Autodesk Inventor part; units mm, degrees
ref_plane "YZ Plane" through (0, 0, 0) normal (1, 0, 0) x (0, 1, 0)
ref_plane "XZ Plane" through (0, 0, 0) normal (0, 1, 0) x (-1, 0, 0)
ref_plane "XY Plane" through (0, 0, 0) normal (0, 0, 1) x (1, 0, 0)
sketch "スケッチ1" plane through (0, 0, 0) normal (0, 1, 0) x (-1, 0, 0)
  line L0 (9.5, -10) -> (-9.5, -10)
  line L1 (-9.5, -10) -> (-9.5, 10)
  line L2 (-9.5, 10) -> (9.5, 10)
  line L3 (9.5, 10) -> (9.5, -10)
  line L4 (9.5, -10) -> (-9.5, 10) construction
  point P0 (0, 0)
  point P1 (0, 0)
  dimension "d0" = 19
  dimension "d1" = 20
extrude "押し出し1" add sketch "スケッチ1" along normal blind 1.5
sketch "スケッチ3" plane through (0, 0, 0) normal (0, -1, 0) x (1, 0, 0)
  line L0 (-9.5, 10) -> (9.5, 10)
  line L1 (-9.5, -10) -> (-9.5, 10)
  line L2 (9.5, -10) -> (-9.5, -10)
  line L3 (9.5, 10) -> (9.5, -10)
  line L4 (-9.5, 0) -> (9.5, 0)
  line L5 (-9.5, 10) -> (9.5, 10)
  line L6 (0, 10) -> (0, -10)
  line L7 (0, 2.5) -> (-3.1667, 2.5)
  line L8 (-3.1667, 2.5) -> (-3.1667, 7.5)
  line L9 (-3.1667, 7.5) -> (0, 7.5)
  line L10 (0, 2.5) -> (3.1667, 2.5)
  line L11 (3.1667, 2.5) -> (3.1667, 7.5)
  line L12 (3.1667, 7.5) -> (0, 7.5)
  line L13 (0, -2.5) -> (-3.1667, -2.5)
  line L14 (-3.1667, -2.5) -> (-3.1667, -7.5)
  line L15 (-3.1667, -7.5) -> (0, -7.5)
  line L16 (3.1667, -2.5) -> (3.1667, -7.5)
  line L17 (0, -2.5) -> (3.1667, -2.5)
  line L18 (3.1667, -7.5) -> (0, -7.5)
  point P0 (0, 0)
  point P1 (0, 0)
  dimension "d8" = 3.1667
  dimension "d9" = 2.5
  dimension "d10" = 5
extrude "押し出し2" add sketch "スケッチ3" along normal blind 1.6 contours L12 L11 L10 L6 | L6 L7 L8 L9 | L17 L16 L18 L6 | L6 L15 L14 L13
sketch "スケッチ4" plane through (0, -1.6, 0) normal (0, -1, 0) x (1, 0, 0)
  line L0 (3.1667, 2.5) -> (3.1667, 7.5)
  line L1 (-3.1667, 7.5) -> (-3.1667, 2.5)
  line L2 (-3.1667, -2.5) -> (-3.1667, -7.5)
  line L3 (3.1667, -7.5) -> (3.1667, -2.5)
  line L4 (3.1667, 7.5) -> (3.1667, 2.5) construction
  line L5 (3.1667, 5) -> (6.3333, 5) construction
  line L6 (6.3333, 5) -> (9.5, 5) construction
  line L7 (9.5, 10) -> (9.5, -10) construction
  line L8 (9.5, 0) -> (-9.5, 0)
  line L9 (-9.5, -10) -> (-9.5, 10)
  line L10 (3.1667, 2.5) -> (-3.1667, 2.5)
  line L11 (0, 2.5) -> (0, -2.5)
  point P0 (0, 0)
  point P1 (6.3333, -5)
  point P2 (-6.3333, 5)
  point P3 (-6.3333, -5)
hole "穴1" at (6.3333, -1.6, 5) at (6.3333, -1.6, -5) at (-6.3333, -1.6, 5) at (-6.3333, -1.6, -5) direction (0, 1, 0) diameter 1.567 end through all
fillet "フィレット1" radius 1.5 8 edges at (3.1667, -0.8, 2.5) (3.1667, -0.8, 7.5) (-3.1667, -0.8, 7.5) (-3.1667, -0.8, 2.5) (3.1667, -0.8, -2.5) (3.1667, -0.8, -7.5) (-3.1667, -0.8, -7.5) (-3.1667, -0.8, -2.5)
properties part number "jump" material "ABS プラスチック"
The listing builds one solid part. Answer for the finished solid, in the listing's coordinates (mm). A direction names the side the tool comes from. Give positions to 0.01 mm unless a question says otherwise; leave off trailing zeros. Write each loop counter-clockwise with the first axis right and the second up, starting at its lowest first coordinate (ties: lowest second). Pieces come first, ordered by that corner, then holes. Notation, with made-up numbers: (-35.75, -4.5) - (21.25, -4.5) arc R23 cw to (21.25, 21.5) - close; hole circle Ø3 at (20.25, 64.5). An arc over 180 degrees is marked (long way). One line per question, with ' | ' between items. Start each with the question number.
1. Straight lines are drawn through the part: line 1 (X direction, y = 0.95, z = 5); line 2 (Z direction, x = -1.75, y = -0.1); line 3 (X direction, y = 0.7, z = 4.5). For each, find the intervals that lie inside material, in ascending order.
2. Section D-D, the plane z = 1 is taken. Determine the outline of the cut face in (x, y), then the cut area to 3 significant figures.
3. Given P1, Ø1.8, axis at y = -0.5, z = 4.5, coming from the +X side; P2, Ø1.8, axis at x = 6.33, z = 5, coming from the -Y side; P3, Ø1.4, axis at x = -6.33, z = -5, coming from the -Y side; P4, Ø0.8, axis at x = 0.5, y = -0.5, coming from the +Z side, each flat-ended and moving along its own axis, determine where each tip first touches the part or whether it passes through.
4. Determine the mould class of faces 1 (the face through (-2.72, -0.81, -2.93)), 2 (the face through (9.5, 1, 0)), 3 (the face through (7.03, 0.76, -5.36)) for opening direction X: +X half, -X half, draft (parallel to the pull), parting line (faces both ways), or undercut.
5. Section A-A, the plane z = -5 is taken. Determine the outline of the cut face in (x, y), then the cut area to 3 significant figures.
6. For faces 4 (the face through (2.74, -0.81, 7.05)), 5 (the face through (2.74, -0.81, -2.95)), 6 (the face through (3.167, -1, -5)), 7 (the face through (-3.167, -1, 5)), determine the directions among +Z, -Z, +X, -X, +Y, -Y from which every point of the face is accessible in a straight line to the end or side of a thin tool.
7. Section C-C, the plane y = 1.1 is taken. Determine the outline of the cut face in (x, z).
8. Section B-B, the plane x = -0.5 is taken. Determine the outline of the cut face in (y, z), then the cut area to 3 significant figures.
Result:
1) line 1: x = -9.5 to -7.12, -5.55 to 5.55, 7.12 to 9.5 | line 2: z = -7.5 to -2.5, 2.5 to 7.5 | line 3: x = -9.5 to -6.94, -5.73 to 5.73, 6.94 to 9.5
2) outline: (-9.5, 0) - (9.5, 0) - (9.5, 1.5) - (-9.5, 1.5) - close | area: 28.5 mm2
3) P1: stops at x = 9.5 | P2: stops at y = 0 | P3: passes through | P4: stops at z = 7.5
4) face 1: -X half | face 2: +X half | face 3: undercut
5) outline: (-9.5, 0) - (-7.12, 0) - (-7.12, 1.5) - (-9.5, 1.5) - close; (-5.55, 0) - (-3.17, 0) - (-3.17, -1.6) - (3.17, -1.6) - (3.17, 0) - (5.55, 0) - (5.55, 1.5) - (-5.55, 1.5) - close; (7.12, 0) - (9.5, 0) - (9.5, 1.5) - (7.12, 1.5) - close | area: 33.9 mm2
6) face 4: +Z, +X, -Y | face 5: +X, -Y | face 6: +Z, -Z, +X, -Y | face 7: +Z, -Z, -X, -Y
7) outline: (-9.5, -10) - (9.5, -10) - (9.5, 10) - (-9.5, 10) - close; hole circle Ø1.57 at (-6.33, -5); hole circle Ø1.57 at (-6.33, 5); hole circle Ø1.57 at (6.33, -5); hole circle Ø1.57 at (6.33, 5)
8) outline: (-1.6, -7.5) - (0, -7.5) - (0, -10) - (1.5, -10) - (1.5, 10) - (0, 10) - (0, 7.5) - (-1.6, 7.5) - (-1.6, 2.5) - (0, 2.5) - (0, -2.5) - (-1.6, -2.5) - close | area: 46.0 mm2
